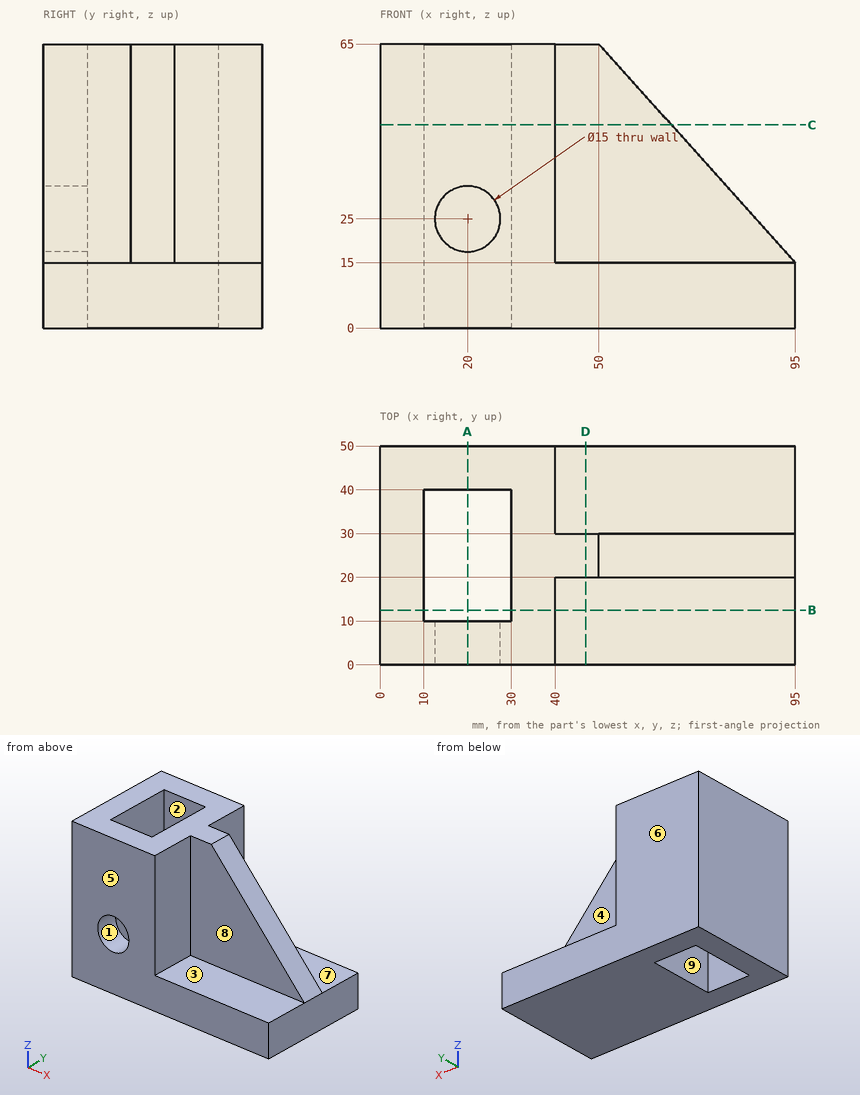
Source: three-view drawing plus pictorial views. Frame: mm from the lowest corner of the part. A direction names the side the tool comes from. Coordinates: 2 decimals unless noted, no trailing zeros. Order: outer loops, then holes, each group sorted by start corner. A loop starts at its lowest first (then second) coordinate and runs counter-clockwise, first axis right, second up. Notation, with made-up numbers: M 42,35 L 46,35 A25 ccw 46,54 Z; hole C 51,21.25 d2. An arc over 180 degrees is marked long. Answer in a Markdown table with one row per item.
(1) Section query A-A, the plane x = 20. Output: boundary loops of the cut face in (y, z), plus the area to 3 significant figures.
Numbers:
| item | result |
|---|---|
| outline | M 0,0 L 10,0 L 10,17.5 L 0,17.5 Z; M 0,32.5 L 10,32.5 L 10,65 L 0,65 Z; M 40,0 L 50,0 L 50,65 L 40,65 Z |
| area | 1,150 mm^2 |
(2) Section query B-B, the plane y = 12.5. Output: boundary loops of the cut face in (x, z), plus the area to 4 significant figures.
Numbers:
| item | result |
|---|---|
| outline | M 0,0 L 10,0 L 10,65 L 0,65 Z; M 30,0 L 95,0 L 95,15 L 40,15 L 40,65 L 30,65 Z |
| area | 2,125 mm^2 |
(3) Section query D-D, the plane x = 47. Output: boundary loops of the cut face in (y, z), plus the area to 3 significant figures.
Numbers:
| item | result |
|---|---|
| outline | M 0,0 L 50,0 L 50,15 L 30,15 L 30,65 L 20,65 L 20,15 L 0,15 Z |
| area | 1,250 mm^2 |
(4) Access query for the marked faces 1, 2, 3, 4 and 5. Directions: +Z, -Z, +X, -X, +Y, -Y. A direction counts if a zero-diameter tool reaches every point of the face in a straight line with its end or side. Return the directions, or none.
Numbers:
| item | result |
|---|---|
| face 1 | -Y |
| face 2 | +Z, -Z |
| face 3 | +Z, +X, -Y |
| face 4 | +Z, +X, +Y |
| face 5 | +Z, -Z, +X, -X, -Y |
(5) Contact query for flat-ended pins moving along their axis: pin 1 Ø10 at (x, z) = (56.5, 28.5) entering from -Y; pin 2 Ø3 at (x, z) = (30, 44) entering from -Y; pin 3 Ø16 at (x, y) = (67.5, 15) entering from +Z; pin 4 Ø16 at (y, z) = (37, 35) entering from +X. Output: stop coordinate, or through.
Numbers:
| item | result |
|---|---|
| pin 1 | stops at y = 20 |
| pin 2 | stops at y = 0 |
| pin 3 | stops at z = 52.49 |
| pin 4 | stops at x = 80.49 |
(6) Section query C-C, the plane z = 46.5. Output: boundary loops of the cut face in (x, y), plus the area to 3 significant figures.
Numbers:
| item | result |
|---|---|
| outline | M 0,0 L 40,0 L 40,20 L 66.65,20 L 66.65,30 L 40,30 L 40,50 L 0,50 Z; hole M 10,10 L 30,10 L 30,40 L 10,40 Z |
| area | 1,670 mm^2 |
(7) Material intervals for line 1 (Z direction, x = 20, y = 5.5); line 2 (Y direction, x = 28, z = 37); line 3 (X direction, y = 34.5, z = 9.5), sorted ascending. Write a range as [from, to].
Numbers:
| item | result |
|---|---|
| line 1 | z = [0, 17.5], [32.5, 65] |
| line 2 | y = [0, 10], [40, 50] |
| line 3 | x = [0, 10], [30, 95] |
(8) Draft query along Y for the marked faces 6, 7, 8 and 9. Return one class per face: pulls with the +Y half, pulls with the -Y half, needs draft (parallel to the pull), parting line crosses it, or undercut.
Numbers:
| item | result |
|---|---|
| face 6 | pulls with the +Y half |
| face 7 | needs draft |
| face 8 | pulls with the -Y half |
| face 9 | undercut |
